Model file for the job. Use its own axes, mm. A direction names the side the tool comes from. Coordinates: 2 decimals unless noted, no trailing zeros. Order: outer loops, then holes, each group sorted by start corner. A loop starts at its lowest first (then second) coordinate and runs counter-clockwise, first axis right, second up. Notation, with made-up numbers: (-5.5, 53.5) - (49.5, 53.5) arc R28 ccw to (49.5, 88.5) - close; hole circle Ø9 at (35, 36.5). An arc over 180 degrees is marked (long way). Put each result on its own line as item: value. Start each with the question number.
```python
from build123d import *

# Parameters (mm, degrees)
F0_W      = 100.234754
F0_H      = 94.90075
F1_DEPTH  = 72.644
F2_W      = 4.22275
F2_H      = 3.333748
F3_DEPTH  = 51.308
F4_W      = 4.222751
F4_H      = 3.111497
F5_DEPTH  = 51.054
F6_W      = 3.778249
F6_H      = 2.666995
F7_DEPTH  = 51.562
F8_W      = 3.333751
F8_H      = 3.111497
F9_DEPTH  = 51.054
F10_W     = 2.666998
F10_H     = 2.222497
F11_DEPTH = 51.562
F12_W     = 2.889253
F12_H     = 2.666999
F13_DEPTH = 51.308
F14_W     = 2.444748
F14_H     = 2.889249
F15_DEPTH = 53.086
F16_W     = 3.333751
F16_H     = 2.889249
F17_DEPTH = 52.578
F18_W     = 3.333751
F18_H     = 2.666998
F19_DEPTH = 51.562


with BuildPart() as f1:
    # F0 (on Top) → F1 (new body)
    with BuildSketch(Plane.XY):
        Rectangle(F0_W, F0_H)
    extrude(amount=F1_DEPTH)

    # F2 (on Front) → F3 (join)
    with BuildSketch(Plane.XZ):
        with Locations((-46.227999, 68.67525)):
            Rectangle(F2_W, F2_H)
    extrude(amount=F3_DEPTH)

    # F4 (on Front) → F5 (join)
    with BuildSketch(Plane.XZ):
        with Locations((-40.227249, 68.786375)):
            Rectangle(F4_W, F4_H)
    extrude(amount=F5_DEPTH)

    # F6 (on Front) → F7 (join)
    with BuildSketch(Plane.XZ):
        with Locations((-34.671002, 69.008626)):
            Rectangle(F6_W, F6_H)
    extrude(amount=F7_DEPTH)

    # F8 (on Front) → F9 (join)
    with BuildSketch(Plane.XZ):
        with Locations((-46.00575, 62.785625)):
            Rectangle(F8_W, F8_H)
    extrude(amount=F9_DEPTH)

    # F10 (on Front) → F11 (join)
    with BuildSketch(Plane.XZ):
        with Locations((-39.893875, 62.785623)):
            Rectangle(F10_W, F10_H)
    extrude(amount=F11_DEPTH)

    # F12 (on Front) → F13 (join)
    with BuildSketch(Plane.XZ):
        with Locations((-34.448751, 62.785623)):
            Rectangle(F12_W, F12_H)
    extrude(amount=F13_DEPTH)

    # F14 (on Front) → F15 (join)
    with BuildSketch(Plane.XZ):
        with Locations((-46.00575, 56.673749)):
            Rectangle(F14_W, F14_H)
    extrude(amount=F15_DEPTH)

    # F16 (on Front) → F17 (join)
    with BuildSketch(Plane.XZ):
        with Locations((-39.782749, 56.451501)):
            Rectangle(F16_W, F16_H)
    extrude(amount=F17_DEPTH)

    # F18 (on Front) → F19 (join)
    with BuildSketch(Plane.XZ):
        with Locations((-34.226501, 56.118125)):
            Rectangle(F18_W, F18_H)
    extrude(amount=F19_DEPTH)


solid = f1.part
```
Item 1: Slice it at B-B, the plane z = 39. Give the cut face in (x, y).
Item 2: Slice it at A-A, the plane x = -4. Give the cut face in (y, z), plus the area to 3 significant figures.
Item 3: Wall check: line 1 along Y through (x, z) = (-41, 12); line 2 along Y through (x, z) = (-35, 55.5). Give the ranges that are in metal, low to high.
Item 4: Pull direction X, two halves, no side cores. Call faces 6 (the face through (-34, -49, 54.785)), 7 (the face through (-42.339, -49, 69)), 8 (the face through (-47.673, -49, 63)), 9 (the face through (-40, -49, 61.674)): pulls with the +X half, pulls with the -X half, needs draft (parallel to the pull), parting line crosses it, or undercut.
Item 5: Flat gauge pins, fed straight in: pin 1 Ø2.5 at (x, z) = (-47, 63.5) entering from -Y; pin 2 Ø0.9 at (y, z) = (-49.5, 62.5) entering from -X; pin 3 Ø2.5 at (y, z) = (-49, 56.5) entering from +X. Where does each tip first touch, or does it go through?
Item 6: 3-axis set-ups, long thin cutter, end or side, ignore diameter. For faces 1 (the face through (-46, -51.308, 69)), 2 (the face through (-46, -49, 61.23)), 3 (the face through (-35, -49, 67.675)), 4 (the face through (-41.45, -50, 56)), 5 (the face through (-38.116, -50, 56)): which of +Z, -Z, +X, -X, +Y, -Y reach the whole face in a straight line?
Here are the results:
1. outline: (-50.12, -47.45) - (50.12, -47.45) - (50.12, 47.45) - (-50.12, 47.45) - close
2. outline: (-47.45, 0) - (47.45, 0) - (47.45, 72.64) - (-47.45, 72.64) - close
2. area: 6,890 mm^2
3. line 1: y = -47.45 to 47.45
3. line 2: y = -51.56 to 47.45
4. face 6: needs draft
4. face 7: undercut
4. face 8: pulls with the -X half
4. face 9: undercut
5. pin 1: stops at y = -51.05
5. pin 2: stops at x = -47.67
5. pin 3: stops at x = -32.56
6. face 1: +Z, -X, -Y
6. face 2: +X, -X, -Y
6. face 3: +X, -Y
6. face 4: -Z, -Y
6. face 5: +Z, -Z, -Y
